Study the drawing (mm; zero at the part's minimum x, y, z) and answer. A direction names the side the tool comes from. Give positions to 0.01 mm unless a question says otherwise; leave off trailing zeros. Order: outer loops, then holes, each group sorted by start corner. A loop starts at its lowest first (then second) coordinate and runs counter-clockwise, first axis right, second up. Notation, with made-up numbers: (0, -8.5) -> (15, -8.5) arc R11 cw to (15, 7.5) -> close; hole circle Ø11 at (29.5, 78). An arc over 180 degrees is marked (long way). Use a Markdown table: item, result. Add a question column.
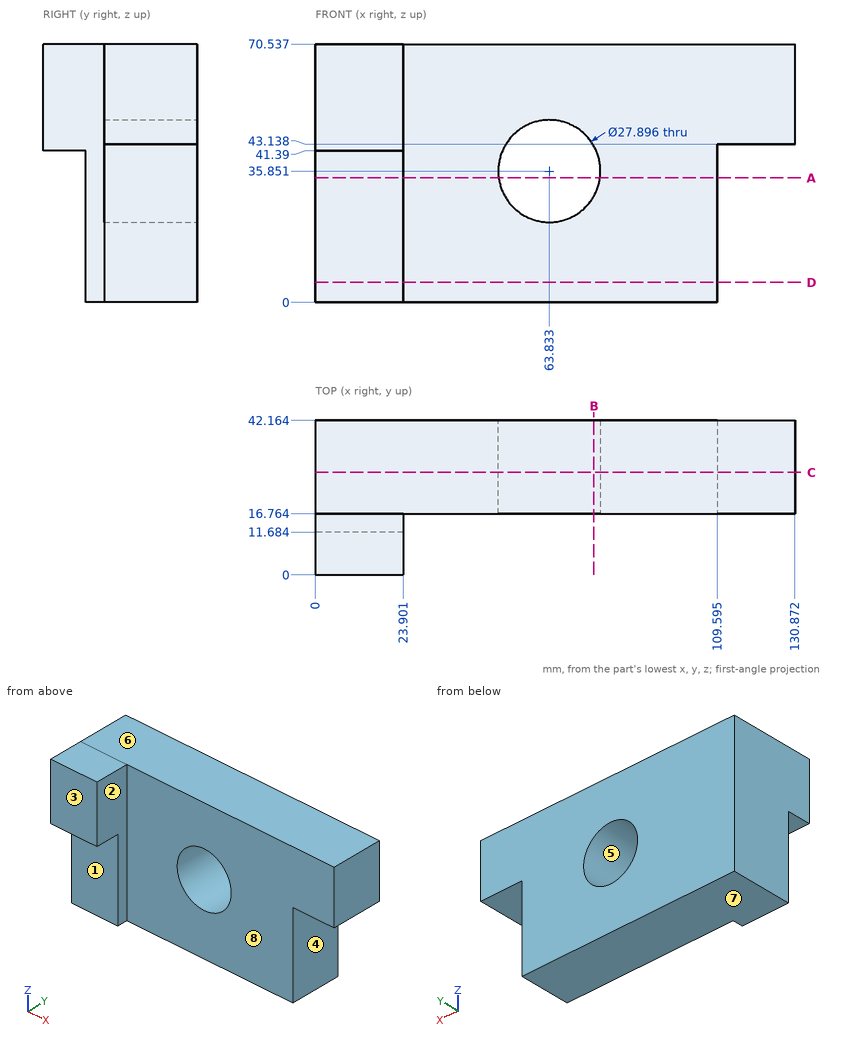
1) The part is cut by section B-B, the plane x = 76. Determine the outline of the cut face in (y, z) (1 decimal), then the cut area to 4 significant figures.
2) The part is cut by section A-A, the plane z = 34. Determine the outline of the cut face in (x, y) (1 decimal).
3) Which of the six approach directions +Z, -Z, +X, -X, +Y, -Y give full straight-line access (tool end or side, diameter ignored) to the marked faces 1, 2, 3 and 4?
4) Straight lines are drawn through the part: line 1 (X direction, y = 37, z = 9) (1 decimal); line 2 (X direction, y = 14, z = 33.5); line 3 (Y direction, x = 35, z = 12.5) (1 decimal). For each, find the intervals that lie inside material, in ascending order.
5) The part is cut by section D-D, the plane z = 5.5. Determine the outline of the cut face in (x, y) (1 decimal), then the cut area to 4 significant figures.
6) Flat-ended cylindrical pins translate along their axes: pin 1 (10.5 mm diameter, centred on x = 120.5, y = 35, fed in from -Z); pin 2 (8.5 mm diameter, centred on y = 12, z = 19, fed in from +X); pin 3 (1 mm diameter, centred on x = 77, z = 41, fed in from -Y); pin 4 (13 mm diameter, centred on x = 16, y = 7, fed in from -Z). Find the tip coordinate at first contact, or state that the pin passes through.
7) Determine the mould class of the marked faces 5, 6, 7 and 8 for opening direction Z: released by +Z, released by -Z, zero draft, split by the parting line, or undercut.
8) The part is cut by section C-C, the plane y = 28. Determine the outline of the cut face in (x, z) (1 decimal), then the cut area to 3 significant figures.
A:
| question | item | result |
|---|---|---|
| 1 | outline | (16.8, 0) -> (42.2, 0) -> (42.2, 29) -> (16.8, 29) -> close; (16.8, 42.7) -> (42.2, 42.7) -> (42.2, 70.5) -> (16.8, 70.5) -> close |
| 1 | area | 1,445 mm^2 |
| 2 | outline | (0, 11.7) -> (23.9, 11.7) -> (23.9, 16.8) -> (50, 16.8) -> (50, 42.2) -> (0, 42.2) -> close; (77.7, 16.8) -> (109.6, 16.8) -> (109.6, 42.2) -> (77.7, 42.2) -> close |
| 3 | face 1 | -Z, +X, -X, -Y |
| 3 | face 2 | +Z, -Z, +X, -Y |
| 3 | face 3 | +Z, -Z, +X, -X, -Y |
| 3 | face 4 | -Z, +X, +Y, -Y |
| 4 | line 1 | 0 to 109.6 |
| 4 | line 2 | 0 to 23.9 |
| 4 | line 3 | 16.8 to 42.2 |
| 5 | outline | (0, 11.7) -> (23.9, 11.7) -> (23.9, 16.8) -> (109.6, 16.8) -> (109.6, 42.2) -> (0, 42.2) -> close |
| 5 | area | 2,905 mm^2 |
| 6 | pin 1 | z = 43.14 |
| 6 | pin 2 | x = 23.9 |
| 6 | pin 3 | y = 16.76 |
| 6 | pin 4 | z = 0 |
| 7 | face 5 | undercut |
| 7 | face 6 | released by +Z |
| 7 | face 7 | released by -Z |
| 7 | face 8 | zero draft |
| 8 | outline | (0, 0) -> (109.6, 0) -> (109.6, 43.1) -> (130.9, 43.1) -> (130.9, 70.5) -> (0, 70.5) -> close; hole circle Ø27.9 at (63.8, 35.9) |
| 8 | area | 7,700 mm^2 |
